Geometry: final body of the model. Coordinates: model frame, mm. A direction names the side the tool comes from. Give positions to 0.01 mm unless a question says otherwise; leave off trailing zeros. Order: outer loops, then holes, each group sorted by start corner. A loop starts at its lowest first (then second) coordinate and runs counter-clockwise, first axis right, second up. Notation, with made-up numbers: (54.25, 33.5) -> (75.25, 33.5) arc R20 cw to (75.25, 64.5) -> close; hole circle Ø5 at (66, 71.5). An arc over 180 degrees is marked (long way). Answer in a Markdown table with one row per item. Add a question column.
Q1. Cut plane A-A on x = 0. Return the cut outline in (y, z).
Q2. Set-up query: faces 5 (the face through (10, 7, 0)), 6 (the face through (10, -7, 0)), 7 (the face through (-9, 0, -1.5)). Return all of +Z, -Z, +X, -X, +Y, -Y with unobstructed straight access to the full face (end or side cutting, diameter ignored); none if empty.
Q3. Cut plane B-B on z = 4.25. Return the cut outline in (x, y).
Q4. Contact query for a flat-ended pin moving along its axis: P1, Ø6, axis at x = 8, y = 8, coming from the -Z side. Output: stop coordinate, or through.
Q5. Line query: line 1 along X through (y, z) = (0, 3); line 2 along X through (y, z) = (1, 2) (3 decimals); line 3 along X through (y, z) = (6.75, 3.5). Output: solid intervals per line, ascending. Write a range as from..to.
Q6. Cut plane D-D on x = 9.5. Return the cut outline in (y, z).
Q7. Pull-direction query (X, two-part tool) for faces 1 (the face through (24.107, -1.081, 1.704)), 2 (the face through (10, -10, 2)), 3 (the face through (-10, 0, 2)), 4 (the face through (13.116, -0.07, 1.704)); classes: +X half, -X half, draft (parallel to the pull), parting line (faces both ways), or undercut.
Q8. Cut plane C-C on y = -2. Return the cut outline in (x, z), and give its area (3 significant figures).
from build123d import *

# Parameters (mm, degrees)
SKETCH_R        = 8.05
PAD_DEPTH       = 5
PAD001_DEPTH    = 40
POCKET_DEPTH    = 1.501
SKETCH002_R     = 1.6
POCKET001_DEPTH = 6.501
FILLET_R        = 3


with BuildPart() as part:
    # Sketch → Pad (new body)
    with BuildSketch(Plane.XY):
        Polygon((-10, 10), (10, 10), (30, 10), (30, -10), (10, -10), (-10, -10), align=None)
        Circle(SKETCH_R, mode=Mode.SUBTRACT)
    extrude(amount=PAD_DEPTH)

    # Sketch001 (on Face3 of Pad) → Pad001 (join)
    with BuildSketch(Plane.YZ.offset(30)):
        Polygon((-4.75, 0), (4.75, 0), (2.95, -1.5), (-2.95, -1.5), align=None)
    extrude(amount=-PAD001_DEPTH)

    # Pad001 Face16 → Pocket (cut, through all)
    with BuildSketch(Plane(origin=(0, 0, 0), x_dir=(0, 1, 0), z_dir=(0, 0, 1))):
        with BuildLine():
            ThreePointArc((-4.75, -6.499231), (-2.498369, -7.652493), (0, -8.05))
            ThreePointArc((0, -8.05), (2.498369, -7.652493), (4.75, -6.499231))
            Line((4.75, -6.499231), (4.75, 6.499231))
            ThreePointArc((4.75, 6.499231), (0, 8.05), (-4.75, 6.499231))
            Line((-4.75, 6.499231), (-4.75, -6.499231))
        make_face()
    extrude(amount=-POCKET_DEPTH, mode=Mode.SUBTRACT)

    # Sketch002 (on Face18 of Pocket) → Pocket001 (cut, through all)
    with BuildSketch(Plane(origin=(0, 0, -1.5), x_dir=(1, 0, 0), z_dir=(0, 0, -1))):
        with Locations((14.714, 0)):
            Circle(SKETCH002_R)
        with Locations((25.286, 0)):
            Circle(SKETCH002_R)
    extrude(amount=-POCKET001_DEPTH, mode=Mode.SUBTRACT)

    # Fillet
    fillet_edges = [part.edges().sort_by_distance(p)[0] for p in [
        (30, -10, 2.5),
        (30, 10, 2.5),
        (-10, -10, 2.5),
        (-10, 10, 2.5),
    ]]
    fillet(fillet_edges, radius=FILLET_R)


solid = part.part
Completed:
| question | item | result |
|---|---|---|
| 1 | outline | (-10, 0) -> (-8.05, 0) -> (-8.05, 5) -> (-10, 5) -> close; (8.05, 0) -> (10, 0) -> (10, 5) -> (8.05, 5) -> close |
| 2 | face 5 | -Z, +X, -X, +Y |
| 2 | face 6 | -Z, +X, -X, -Y |
| 2 | face 7 | -Z, +X, -X, +Y, -Y |
| 3 | outline | (-10, -7) arc R3 ccw to (-7, -10) -> (27, -10) arc R3 ccw to (30, -7) -> (30, 7) arc R3 ccw to (27, 10) -> (-7, 10) arc R3 ccw to (-10, 7) -> close; hole circle Ø16.1 at (0, 0); hole circle Ø3.2 at (14.71, 0); hole circle Ø3.2 at (25.29, 0) |
| 4 | P1 | stops at z = 0 |
| 5 | line 1 | x = -10..-8.05, 8.05..13.11, 16.31..23.69, 26.89..30 |
| 5 | line 2 | x = -10..-7.988, 7.988..13.465, 15.963..24.037, 26.535..30 |
| 5 | line 3 | x = -10..-4.39, 4.39..30 |
| 6 | outline | (-10, 0) -> (-4.75, 0) -> (-2.95, -1.5) -> (2.95, -1.5) -> (4.75, 0) -> (10, 0) -> (10, 5) -> (-10, 5) -> close |
| 7 | face 1 | undercut |
| 7 | face 2 | draft |
| 7 | face 3 | -X half |
| 7 | face 4 | undercut |
| 8 | outline | (-10, -1.5) -> (-7.8, -1.5) -> (-7.8, 5) -> (-10, 5) -> close; (7.8, -1.5) -> (30, -1.5) -> (30, 5) -> (7.8, 5) -> close |
| 8 | area | 159 mm² |
